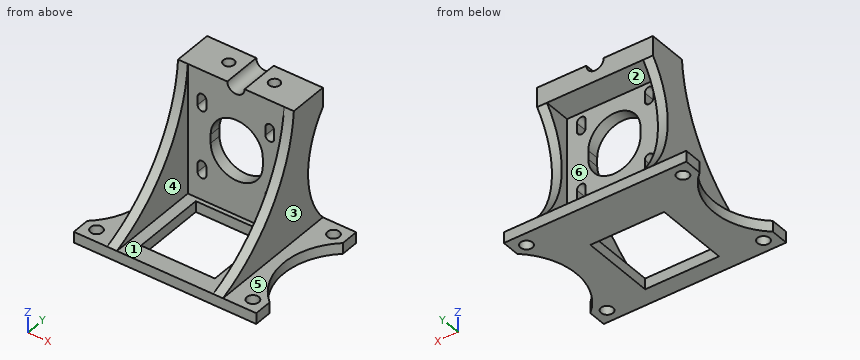
```python
from build123d import *

# Parameters (mm, degrees)
SKETCH2_R                = 2.75
SKETCH2_W                = 34
SKETCH2_H                = 34
BOSS_EXTRUDE1_DEPTH      = 5
SKETCH3_W                = 4.5
SKETCH3_H                = 44
SKETCH3_H_2              = 18
SKETCH3_W_2              = 44.3
BOSS_EXTRUDE2_DEPTH      = 60
CUT_EXTRUDE1_DEPTH       = 16.35
CUT_EXTRUDE1_DEPTH_BACK  = 60
CUT_EXTRUDE3_DEPTH       = 16.35
CUT_EXTRUDE3_DEPTH_BACK  = 60
CUT_EXTRUDE6_REACH       = 25.5
CUT_EXTRUDE6_START       = -5.5
SKETCH9_W                = 44.3
SKETCH9_H                = 51
CUT_EXTRUDE7_DEPTH       = 5.5
LPATTERN1_COUNT          = 2
LPATTERN1_PITCH          = 31.25
LPATTERN2_COUNT          = 2
LPATTERN2_PITCH          = 31
LPATTERN2_COPY_1_DEPTH   = 5.5
CUT_EXTRUDE8_DEPTH       = 10
CUT_EXTRUDE10_DEPTH      = 45
CUT_EXTRUDE10_DEPTH_BACK = 19
SKETCH15_R               = 2.5
CUT_EXTRUDE11_DEPTH      = 4.6
LPATTERN3_COUNT          = 2
LPATTERN3_PITCH          = 21


with BuildPart() as part:
    # Sketch2 → Boss-Extrude1 (new body)
    with BuildSketch(Plane.XY):
        with BuildLine():
            Line((0, -53.68), (0, -62))
            Line((0, -62), (84, -62))
            Line((84, -62), (84, -53.68))
            ThreePointArc((84, -53.68), (73.637148469, -31), (84, -8.32))
            Line((84, -8.32), (84, 0))
            Line((84, 0), (0, 0))
            Line((0, 0), (0, -8.32))
            ThreePointArc((0, -8.32), (10.362851531, -31), (0, -53.68))
        make_face()
        with Locations((6, -6)):
            Circle(SKETCH2_R, mode=Mode.SUBTRACT)
        with Locations((78, -56)):
            Circle(SKETCH2_R, mode=Mode.SUBTRACT)
        with Locations((6, -56)):
            Circle(SKETCH2_R, mode=Mode.SUBTRACT)
        with Locations((78, -6)):
            Circle(SKETCH2_R, mode=Mode.SUBTRACT)
        with Locations((42, -37)):
            Rectangle(SKETCH2_W, SKETCH2_H, mode=Mode.SUBTRACT)
    extrude(amount=BOSS_EXTRUDE1_DEPTH)

    # Sketch3 → Boss-Extrude2 (add)
    with BuildSketch(Plane.XY.offset(5)):
        with Locations((17.6, -40)):
            Rectangle(SKETCH3_W, SKETCH3_H)
        with Locations((66.4, -40)):
            Rectangle(SKETCH3_W, SKETCH3_H)
        with Locations((66.4, -9)):
            Rectangle(SKETCH3_W, SKETCH3_H_2)
        with Locations((17.6, -9)):
            Rectangle(SKETCH3_W, SKETCH3_H_2)
        with Locations((42, -9)):
            Rectangle(SKETCH3_W_2, SKETCH3_H_2)
    extrude(amount=BOSS_EXTRUDE2_DEPTH)

    # Sketch6 → Cut-Extrude1 (cut, two sides)
    with BuildSketch(Plane(origin=(68.65, 0, 0), x_dir=(0, 0, -1), z_dir=(1, 0, 0))) as cut_extrude1_sk:
        with BuildLine():
            Line((62.328372383, -231.688052054), (-5, -62))
            ThreePointArc((-5, -62), (-28.669965475, -31.368134738), (-65, -18))
            Line((-65, -18), (-247.078635565, -4.789579558))
            Line((-247.078635565, -4.789579558), (-462.994068413, -299.219715259))
            Line((-462.994068413, -299.219715259), (-153.587060464, -526.118187755))
            Line((-153.587060464, -526.118187755), (62.328372383, -231.688052054))
        make_face()
    extrude(amount=CUT_EXTRUDE1_DEPTH, mode=Mode.SUBTRACT)
    extrude(cut_extrude1_sk.sketch, amount=-CUT_EXTRUDE1_DEPTH_BACK, mode=Mode.SUBTRACT)

    # Sketch7 → Cut-Extrude3 (cut, two sides)
    with BuildSketch(Plane(origin=(68.65, 0, 0), x_dir=(0, 0, -1), z_dir=(1, 0, 0))) as cut_extrude3_sk:
        with BuildLine():
            ThreePointArc((-56, 0), (-30.5, -9.181985788), (-5, 0))
            Line((-5, 0), (-56, 0))
        make_face()
    extrude(amount=CUT_EXTRUDE3_DEPTH, mode=Mode.SUBTRACT)
    extrude(cut_extrude3_sk.sketch, amount=-CUT_EXTRUDE3_DEPTH_BACK, mode=Mode.SUBTRACT)

    # Sketch9 → Cut-Extrude6 (cut, up to next)
    with BuildSketch(Plane.XZ.offset(18).offset(CUT_EXTRUDE6_START), mode=Mode.PRIVATE) as cut_extrude6_sk1:
        with Locations((42, 30.5)):
            Rectangle(SKETCH9_W, SKETCH9_H)
    cut_extrude6_tool1 = extrude(cut_extrude6_sk1.sketch, amount=-CUT_EXTRUDE6_REACH, mode=Mode.PRIVATE) & part.part
    add(cut_extrude6_tool1.solids().sort_by_distance((42, -12.5, 30.5))[0], mode=Mode.SUBTRACT)

    # Sketch10 → Cut-Extrude7 (cut)
    with BuildSketch(Plane(origin=(0, -12.5, 0), x_dir=(1, 0, 0), z_dir=(0, 1, 0))):
        with BuildLine():
            Line((28.35, -17), (28.35, -21))
            ThreePointArc((28.35, -21), (26.35, -23), (24.35, -21))
            Line((24.35, -21), (24.35, -17))
            ThreePointArc((24.35, -17), (26.35, -15), (28.35, -17))
        make_face()
    cut_extrude7 = extrude(amount=-CUT_EXTRUDE7_DEPTH, mode=Mode.SUBTRACT)

    # LPattern1: Cut-Extrude7 ×2
    with Locations(*[(i * LPATTERN1_PITCH, 0, 0) for i in range(1, LPATTERN1_COUNT)]):
        add(cut_extrude7, mode=Mode.SUBTRACT)

    # LPattern2: Cut-Extrude7 ×2
    with Locations(*[(0, 0, i * LPATTERN2_PITCH) for i in range(1, LPATTERN2_COUNT)]):
        add(cut_extrude7, mode=Mode.SUBTRACT)

    # LPattern2 copy 1 sketch → LPattern2 copy 1 (cut)
    with BuildSketch(Plane(origin=(31.25, -12.5, 31), x_dir=(1, 0, 0), z_dir=(0, 1, 0))):
        with BuildLine():
            Line((28.35, -17), (28.35, -21))
            ThreePointArc((28.35, -21), (26.35, -23), (24.35, -21))
            Line((24.35, -21), (24.35, -17))
            ThreePointArc((24.35, -17), (26.35, -15), (28.35, -17))
        make_face()
    extrude(amount=-LPATTERN2_COPY_1_DEPTH, mode=Mode.SUBTRACT)

    # Sketch11 → Cut-Extrude8 (cut)
    with BuildSketch(Plane(origin=(0, -12.5, 0), x_dir=(1, 0, 0), z_dir=(0, 1, 0))):
        with BuildLine():
            Line((54.35, -33), (54.35, -37))
            ThreePointArc((54.35, -37), (42.35, -49), (30.35, -37))
            Line((30.35, -37), (30.35, -33))
            ThreePointArc((30.35, -33), (42.35, -21), (54.35, -33))
        make_face()
    extrude(amount=-CUT_EXTRUDE8_DEPTH, mode=Mode.SUBTRACT)

    # Sketch14 → Cut-Extrude10 (cut, two sides)
    with BuildSketch(Plane.XZ.offset(18)) as cut_extrude10_sk:
        with BuildLine():
            Line((38, 234.260792413), (38, 65))
            ThreePointArc((38, 65), (42, 61), (46, 65))
            Line((46, 65), (46, 234.260792413))
            Line((46, 234.260792413), (46, 572.782377239))
            Line((46, 572.782377239), (38, 572.782377239))
            Line((38, 572.782377239), (38, 234.260792413))
        make_face()
    extrude(amount=CUT_EXTRUDE10_DEPTH, mode=Mode.SUBTRACT)
    extrude(cut_extrude10_sk.sketch, amount=-CUT_EXTRUDE10_DEPTH_BACK, mode=Mode.SUBTRACT)

    # Sketch15 → Cut-Extrude11 (cut)
    with BuildSketch(Plane.XY.offset(65)):
        with Locations((31.5, -8.25)):
            Circle(SKETCH15_R)
    cut_extrude11 = extrude(amount=-CUT_EXTRUDE11_DEPTH, mode=Mode.SUBTRACT)

    # LPattern3: Cut-Extrude11 ×2
    with Locations(*[(i * LPATTERN3_PITCH, 0, 0) for i in range(1, LPATTERN3_COUNT)]):
        add(cut_extrude11, mode=Mode.SUBTRACT)


solid = part.part
```
The listing builds one solid part. Answer for the finished solid, in the listing's coordinates (mm). Face numbers are marked on the shaded views. A direction names the side the tool comes from. Coordinates: 2 decimals unless noted, no trailing zeros. Write each loop counter-clockwise with the first axis right and the second up, starting at its lowest first coordinate (ties: lowest second). Pieces come first, ordered by that corner, then holes. Notation, with made-up numbers: (25.5, 52.25) - (51.5, 52.25) arc R22 cw to (51.5, 68.25) - close; hole circle Ø5 at (85, -27.75). An arc over 180 degrees is marked (long way). Return JSON: item names as keys, results as strings. Group by question number.
Q1. The part is cut by section B-B on y = -56. Write down the section's boundary in (x, z).
Q2. The part is cut by section C-C on x = 42.35. Write down the section's boundary in (y, z).
Q3. Which of the six approach directions +Z, -Z, +X, -X, +Y, -Y give full straight-line access (tool end or side, diameter ignored) to the marked faces 1, 2 and 3?
Q4. For a pull along Z with two mould halves and no side action, classify the marked faces 4, 5 and 6 as +Z half, -Z half, draft (parallel to the pull), parting line (faces both ways), or undercut.
Q5. The part is cut by section A-A on x = 26.35. Write down the section's boundary in (y, z), and give its area (4 significant figures).
Q6. The part is cut by section D-D on z = 45. Write down the section's boundary in (x, y), and give its area (3 significant figures).
Q7. Find the intervals of material crossed by line 1 along X through (y, z) = (-36.5, 11.5); line 2 along Y through (x, z) = (6, 3.45); line 3 along X through (y, z) = (-8, 64), in increasing order. Write a range as [from, to].
Q8. Flat-ended cylindrical pins translate along their axes: pin 1 Ø4.5 at (y, z) = (-16, 19) entering from -X; pin 2 Ø22 at (x, z) = (48, 38) entering from +Y; pin 3 Ø5.5 at (y, z) = (-37.5, 3.5) entering from +X. Find the tip coordinate at first contact, or state that the pin passes through.
Evaluation:
{
 "1": {"outline": "(0, 0) - (3.25, 0) - (3.25, 5) - (0, 5) - close; (8.75, 0) - (75.25, 0) - (75.25, 5) - (68.65, 5) - (68.65, 7.71) - (64.15, 7.71) - (64.15, 5) - (19.85, 5) - (19.85, 7.71) - (15.35, 7.71) - (15.35, 5) - (8.75, 5) - close; (80.75, 0) - (84, 0) - (84, 5) - (80.75, 5) - close"},
 "2": {"outline": "(-62, 0) - (-54, 0) - (-54, 5) - (-62, 5) - close; (-20, 0) - (0, 0) - (0, 5) - (-12.5, 5) - (-12.5, 21) - (-18, 21) - (-18, 5) - (-20, 5) - close; (-18, 49) - (-12.5, 49) - (-12.5, 56) - (0, 56) - (0, 61.02) - (-18, 61.02) - close"},
 "3": {"face 1": "+Z, -Y", "face 2": "+Y", "face 3": "+Z, +X, +Y, -Y"},
 "4": {"face 4": "draft", "face 5": "+Z half", "face 6": "undercut"},
 "5": {"outline": "(-62, 0) - (-54, 0) - (-54, 5) - (-62, 5) - close; (-20, 0) - (0, 0) - (0, 5) - (-12.5, 5) - (-12.5, 15) - (-18, 15) - (-18, 5) - (-20, 5) - close; (-18, 23) - (-12.5, 23) - (-12.5, 46) - (-18, 46) - close; (-18, 54) - (-12.5, 54) - (-12.5, 56) - (0, 56) - (0, 65) - (-18, 65) - close", "area": "494.5 mm2"},
 "6": {"outline": "(15.35, -22.46) - (19.85, -22.46) - (19.85, -18) - (33.41, -18) - (33.41, -12.5) - (19.85, -12.5) - (19.85, -6.46) - (15.35, -6.46) - close; (51.29, -18) - (64.15, -18) - (64.15, -22.46) - (68.65, -22.46) - (68.65, -6.46) - (64.15, -6.46) - (64.15, -12.5) - (51.29, -12.5) - close", "area": "289 mm2"},
 "7": {"line 1": "x = [15.35, 19.85], [64.15, 68.65]", "line 2": "y = [-62, -58.75], [-53.25, -46.58], [-15.42, -8.75], [-3.25, 0]", "line 3": "x = [15.35, 29.01], [33.99, 38.13], [45.87, 50.01], [54.99, 68.65]"},
 "8": {"pin 1": "stops at x = 15.35", "pin 2": "stops at y = -12.5", "pin 3": "stops at x = 75.1"}
}
